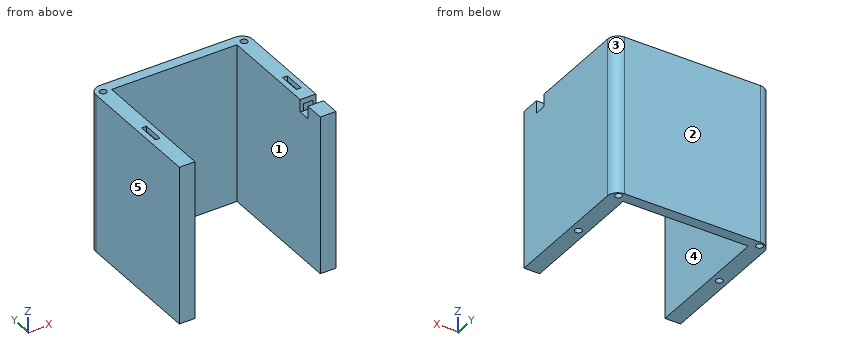
from build123d import *

# Parameters (mm, degrees)
SKETCH2_W           = 120
SKETCH2_H           = 114.5
BOSS_EXTRUDE1_DEPTH = 152
SKETCH3_R           = 3.25
CUT_EXTRUDE1_DEPTH  = 27.5
SKETCH4_W           = 120
SKETCH4_H           = 10.090135052
CUT_EXTRUDE2_DEPTH  = 192.859758942
SKETCH5_W           = 9.929816524
SKETCH5_H           = 99.5
SKETCH5_W_2         = 106.146314573
SKETCH5_H_2         = 4.565432885
SKETCH5_W_3         = 9.245001591
CUT_EXTRUDE3_DEPTH  = 140
SKETCH6_W           = 5
SKETCH6_H           = 99.5
BOSS_EXTRUDE2_DEPTH = 10
SKETCH7_W           = 106.146314573
SKETCH7_H           = 5
BOSS_EXTRUDE3_DEPTH = 6
SKETCH8_W           = 5
SKETCH8_H           = 99.5
BOSS_EXTRUDE4_DEPTH = 10
SKETCH9_R           = 3.25
CUT_EXTRUDE4_DEPTH  = 5
SKETCH11_W          = 12
SKETCH11_H          = 11.501568892
CUT_EXTRUDE5_DEPTH  = 35
SKETCH12_W          = 6.942410631
SKETCH12_H          = 9.961568892
BOSS_EXTRUDE5_DEPTH = 9.5
SKETCH13_W          = 4.5
SKETCH13_H          = 20.5
CUT_EXTRUDE6_DEPTH  = 15


with BuildPart() as part:
    # Sketch2 → Boss-Extrude1 (new body)
    with BuildSketch(Plane.XY):
        with BuildLine():
            Line((-48.742911668, 61.163031625), (81.257088332, 61.163031625))
            ThreePointArc((81.257088332, 61.163031625), (88.328156143, 58.234099437), (91.257088332, 51.163031625))
            Line((91.257088332, 51.163031625), (91.257088332, -73.336968375))
            Line((91.257088332, -73.336968375), (-58.742911668, -73.336968375))
            Line((-58.742911668, -73.336968375), (-58.742911668, 51.163031625))
            ThreePointArc((-58.742911668, 51.163031625), (-55.81397948, 58.234099437), (-48.742911668, 61.163031625))
        make_face()
        with Locations((16.257088332, -6.086968375)):
            Rectangle(SKETCH2_W, SKETCH2_H, mode=Mode.SUBTRACT)
    extrude(amount=BOSS_EXTRUDE1_DEPTH)

    # Sketch3 → Cut-Extrude1 (cut)
    with BuildSketch(Plane.XY.offset(152)):
        with Locations((-51.242911668, 52.163031625)):
            Circle(SKETCH3_R)
        with Locations(Location((83.757088332, 52.163031625, 0), (0, 0, 180))):
            Circle(SKETCH3_R)
    extrude(amount=-CUT_EXTRUDE1_DEPTH, mode=Mode.SUBTRACT)

    # Sketch4 → Cut-Extrude2 (cut, through all)
    with BuildSketch(Plane.XY.offset(152)):
        with Locations((16.257088332, -68.382035901)):
            Rectangle(SKETCH4_W, SKETCH4_H)
    extrude(amount=-CUT_EXTRUDE2_DEPTH, mode=Mode.SUBTRACT)

    # Sketch5 → Cut-Extrude3 (cut)
    with BuildSketch(Plane.XY.offset(152)):
        with Locations((-51.653725831, -3.586968375)):
            Rectangle(SKETCH5_W, SKETCH5_H)
        with Locations((16.314156243, 56.459462148)):
            Rectangle(SKETCH5_W_2, SKETCH5_H_2)
        with Locations((83.825495028, -3.586968375)):
            Rectangle(SKETCH5_W_3, SKETCH5_H)
    extrude(amount=-CUT_EXTRUDE3_DEPTH, mode=Mode.SUBTRACT)

    # Sketch6 → Boss-Extrude2 (add)
    with BuildSketch(Plane.ZY.offset(46.688817569)):
        with Locations((149.5, -3.586968375)):
            Rectangle(SKETCH6_W, SKETCH6_H)
    extrude(amount=BOSS_EXTRUDE2_DEPTH)

    # Sketch7 → Boss-Extrude3 (add)
    with BuildSketch(Plane(origin=(0, 54.176745705, 0), x_dir=(1, 0, 0), z_dir=(0, 1, 0))):
        with Locations((16.314156243, -149.5)):
            Rectangle(SKETCH7_W, SKETCH7_H)
    extrude(amount=BOSS_EXTRUDE3_DEPTH)

    # Sketch8 → Boss-Extrude4 (add)
    with BuildSketch(Plane(origin=(79.202994232, 0, 0), x_dir=(0, 0, -1), z_dir=(1, 0, 0))):
        with Locations((-149.5, -3.586968375)):
            Rectangle(SKETCH8_W, SKETCH8_H)
    extrude(amount=BOSS_EXTRUDE4_DEPTH)

    # Sketch9 → Cut-Extrude4 (cut)
    with BuildSketch(Plane(origin=(0, 0, 0), x_dir=(-1, 0, 0), z_dir=(0, 0, -1))):
        with Locations((-83.757088332, 56.163031625)):
            Circle(SKETCH9_R)
        with Locations((-83.757088332, -3.836968375)):
            Circle(SKETCH9_R)
        with Locations(Location((51.242911668, -3.836968375, 0), (0, 0, 180))):
            Circle(SKETCH9_R)
        with Locations(Location((51.242911668, 56.163031625, 0), (0, 0, 180))):
            Circle(SKETCH9_R)
    extrude(amount=-CUT_EXTRUDE4_DEPTH, mode=Mode.SUBTRACT)

    # Sketch11 → Cut-Extrude5 (cut)
    with BuildSketch(Plane(origin=(91.257088332, 0, 0), x_dir=(0, 0, -1), z_dir=(1, 0, 0))):
        with Locations((-146, -49.126183929)):
            Rectangle(SKETCH11_W, SKETCH11_H)
    extrude(amount=-CUT_EXTRUDE5_DEPTH, mode=Mode.SUBTRACT)

    # Sketch12 → Boss-Extrude5 (add)
    with BuildSketch(Plane(origin=(79.202994232, 0, 0), x_dir=(0, 0, -1), z_dir=(1, 0, 0))):
        with Locations((-136.528794684, -48.356183929)):
            Rectangle(SKETCH12_W, SKETCH12_H)
    extrude(amount=BOSS_EXTRUDE5_DEPTH)

    # Sketch13 → Cut-Extrude6 (cut)
    with BuildSketch(Plane.XY.offset(152)):
        with Locations((83.757088332, -19.086968375)):
            Rectangle(SKETCH13_W, SKETCH13_H)
        with Locations((-51.242911668, -19.086968375)):
            Rectangle(SKETCH13_W, SKETCH13_H)
    extrude(amount=-CUT_EXTRUDE6_DEPTH, mode=Mode.SUBTRACT)


solid = part.part
Source: CAD feature listing. Evaluate the final solid. Frame: model axes, mm. Face numbers are marked on the shaded views. A direction names the side the tool comes from. Give positions to 0.01 mm unless a question says otherwise; leave off trailing zeros. Write each loop counter-clockwise with the first axis right and the second up, starting at its lowest first coordinate (ties: lowest second). Pieces come first, ordered by that corner, then holes. Notation, with made-up numbers: (-16.5, 58) -> (11.5, 58) arc R23 ccw to (11.5, 71) -> close; hole circle Ø7 at (76.25, 82). An arc over 180 degrees is marked (long way). Return JSON: item names as keys, results as strings. Group by question number.
1. Section A-A, the plane y = 41. Output: boundary loops of the cut face in (x, z).
2. Pin query (flat end, axial travel): pin 1 Ø2 at (x, y) = (-51, -5) entering from -Z; pin 2 Ø5 at (x, y) = (-50.5, 55) entering from -Z; pin 3 Ø2 at (x, z) = (8, 123.5) entering from -Y; pin 4 Ø2.5 at (y, z) = (55.5, 107) entering from -X. Return the tip coordinate at first contact, or that it passes through.
3. Section C-C, the plane y = -23. Output: boundary loops of the cut face in (x, z), then the cut area to 3 significant figures.
4. Material intervals for line 1 (X direction, y = 33, z = 47); line 2 (Y direction, x = 3.5, z = 91.5); line 3 (Z direction, x = 56, y = 55.5), sorted ascending. Write a range as from..to.
5. Section D-D, the plane x = -27.5. Output: boundary loops of the cut face in (y, z), then the cut area to 3 significant figures.
6. Mould query, pull axis X, two halves, no side actions, for the marked faces 3, 4 and 5. Classes: +X half, -X half, draft (parallel to the pull), parting line (faces both ways), or undercut.
7. Access query for the marked faces 1 and 2. Directions: +Z, -Z, +X, -X, +Y, -Y. A direction counts if a zero-diameter tool reaches every point of the face in a straight line with its end or side. Return the directions, or none.
8. Section B-B, the plane z = 87. Output: boundary loops of the cut face in (x, y).
Determined:
{
 "1": {"outline": "(-58.74, 0) -> (-43.74, 0) -> (-43.74, 152) -> (-58.74, 152) -> close; (76.26, 0) -> (91.26, 0) -> (91.26, 152) -> (76.26, 152) -> close; hole (-56.62, 12) -> (-46.69, 12) -> (-46.69, 147) -> (-56.62, 147) -> close; hole (79.2, 12) -> (88.45, 12) -> (88.45, 147) -> (79.2, 147) -> close"},
 "2": {"pin 1": "stops at z = 5", "pin 2": "stops at z = 0", "pin 3": "stops at y = 51.16", "pin 4": "stops at x = -58.25"},
 "3": {"outline": "(-58.74, 0) -> (-43.74, 0) -> (-43.74, 152) -> (-48.99, 152) -> (-48.99, 147) -> (-46.69, 147) -> (-46.69, 12) -> (-56.62, 12) -> (-56.62, 147) -> (-53.49, 147) -> (-53.49, 152) -> (-58.74, 152) -> close; (76.26, 0) -> (91.26, 0) -> (91.26, 152) -> (86.01, 152) -> (86.01, 147) -> (88.45, 147) -> (88.45, 12) -> (79.2, 12) -> (79.2, 147) -> (81.51, 147) -> (81.51, 152) -> (76.26, 152) -> close", "area": "1,930 mm2"},
 "4": {"line 1": "x = -58.74..-56.62, -46.69..-43.74, 76.26..79.2, 88.45..91.26", "line 2": "y = 51.16..54.18, 58.74..61.16", "line 3": "z = 0..12, 147..152"},
 "5": {"outline": "(51.16, 0) -> (61.16, 0) -> (61.16, 152) -> (51.16, 152) -> close; hole (54.18, 12) -> (58.74, 12) -> (58.74, 147) -> (54.18, 147) -> close", "area": "904 mm2"},
 "6": {"face 3": "+X half", "face 4": "undercut", "face 5": "-X half"},
 "7": {"face 1": "+Z, -Z, -Y", "face 2": "+Z, -Z, +X, -X, +Y"},
 "8": {"outline": "(-58.74, -73.34) -> (-43.74, -73.34) -> (-43.74, 51.16) -> (76.26, 51.16) -> (76.26, -73.34) -> (91.26, -73.34) -> (91.26, 51.16) arc R10 ccw to (81.26, 61.16) -> (-48.74, 61.16) arc R10 ccw to (-58.74, 51.16) -> close; hole (-56.62, -53.34) -> (-46.69, -53.34) -> (-46.69, 46.16) -> (-56.62, 46.16) -> close; hole (-36.76, 54.18) -> (69.39, 54.18) -> (69.39, 58.74) -> (-36.76, 58.74) -> close; hole (79.2, -53.34) -> (88.45, -53.34) -> (88.45, 46.16) -> (79.2, 46.16) -> close"}
}
